Input: dimensioned drawing with shaded views. Units: mm. Origin: part minimum x, y, z. Give positions to 0.01 mm unless a question says otherwise; leave off trailing zeros. Loops run counter-clockwise (first coordinate to the right, second up) from the corner with the lowest first, then second, coordinate; pieces in that order, holes last.
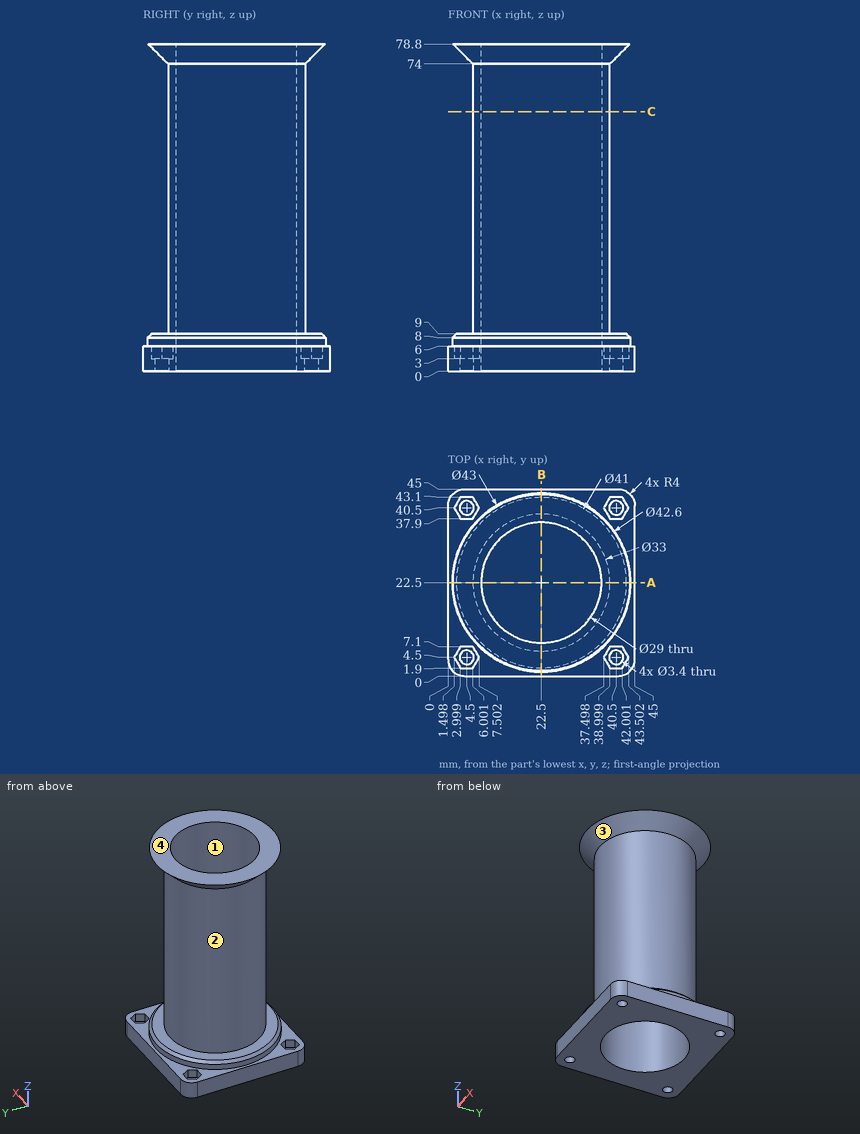
(1) First-contact query: pin 1 (5 mm diameter, centred on x = 19, z = 50.5, fed in from -Y); pin 2 (5.5 mm diameter, centred on x = 40.5, y = 40, fed in from +Z); pin 3 (10 mm diameter, centred on y = 9.5, z = 14.5, fed in from +X). Flat tips, straight axial feed; report the tip coordinate or a pass-through.
A:
pin 1: stops at y = 6.03
pin 2: stops at z = 6
pin 3: stops at x = 36.93
(2) Section C-C, the plane z = 62.5. Return the cut outline in (x, y), then the cut area to 3 significant figures.
A:
outline: circle Ø33 at (22.5, 22.5); hole circle Ø29 at (22.5, 22.5)
area: 195 mm2
(3) Mould query, pull axis Z, two halves, no side actions, for the marked faces 1, 2, 3 and 4. Classes: pulls with the +Z half, pulls with the -Z half, needs draft (parallel to the pull), parting line crosses it, or undercut.
A:
face 1: needs draft
face 2: undercut
face 3: undercut
face 4: pulls with the +Z half
(4) Ray query, line 1 along Y through (x, z) = (40.5, 2.25); line 2 along Y through (x, z) = (22, 36); line 3 along Y through (x, z) = (40, 1) (1 decimal). Return the intervals inside material, ascending.
A:
line 1: y = 0 to 2.8, 6.2 to 38.8, 42.2 to 45
line 2: y = 6.01 to 8.01, 36.99 to 38.99
line 3: y = 0 to 2.9, 6.1 to 38.9, 42.1 to 45
(5) Section A-A, the plane y = 22.5. Return the cut outline in (x, z), then the cut area to 3 significant figures.
A:
outline: (0, 0) - (8, 0) - (8, 78.8) - (1.2, 78.8) - (6, 74) - (6, 9) - (2, 9) - (1, 8) - (1, 6) - (0, 6) - close; (37, 0) - (45, 0) - (45, 6) - (44, 6) - (44, 8) - (43, 9) - (39, 9) - (39, 74) - (43.8, 78.8) - (37, 78.8) - close
area: 439 mm2
